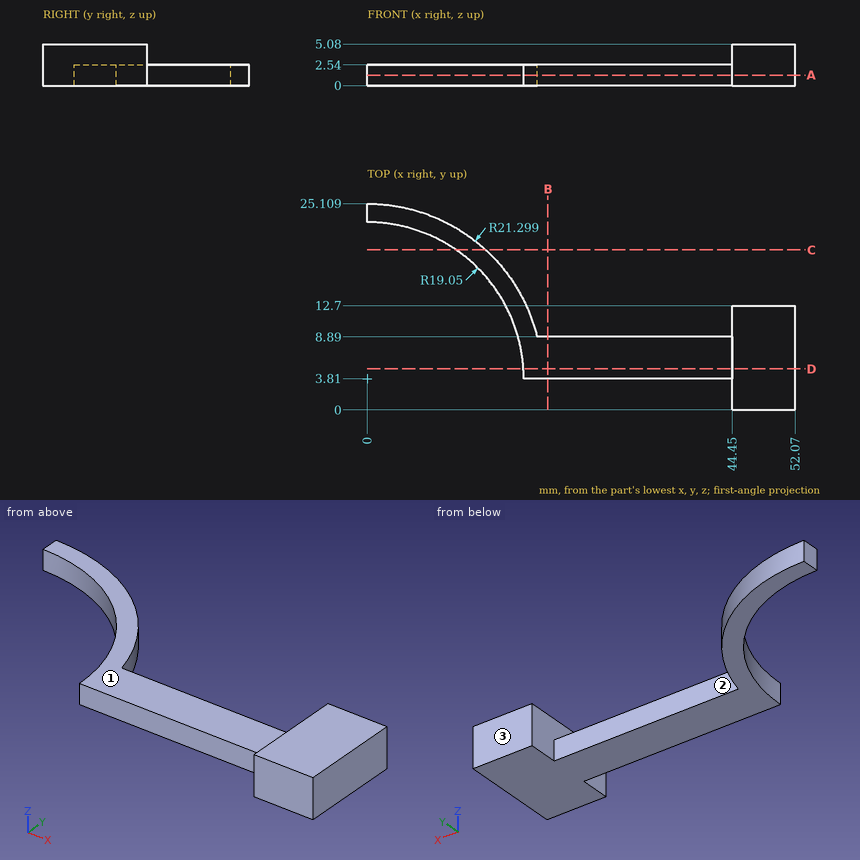
The figure shows three views and two pictorial views of one solid part (mm, origin at its lowest corner). Answer the questions. A direction names the side the tool comes from. Coordinates: 2 decimals unless noted, no trailing zeros. Loops run counter-clockwise (first coordinate to the right, second up) from the corner with the lowest first, then second, coordinate; pieces in that order, holes last. Notation, with made-up numbers: M 71.5,35 L 85.5,35 A31 ccw 85.5,59 Z; hole C 66,-32 d8. An arc over 180 degrees is marked long. Use CSV: the item, a comma, the result in double quotes. Start each with the question number.
(1) Given pin 1 Ø1.3 at (x, z) = (38, 2) entering from -Y; pin 2 Ø1 at (y, z) = (14, 2.5) entering from -X; pin 3 Ø3 at (y, z) = (21, 2) entering from +X (1 decimal), each flat-ended and moving along its own axis, determine where each tip first touches the part or whether it passes through.
(2) Find section C-C, the plane y = 19.5. Give the vertices of the cut face in (x, z).
(3) For the marked faces 1, 2 and 3, determine the directions among +Z, -Z, +X, -X, +Y, -Y from which every point of the face is accessible in a straight line to the end or side of a thin tool.
(4) Consider line 1 (Y direction, x = 35, z = 0.35); line 2 (X direction, y = 11.75, z = 4.1); line 3 (Z direction, x = 31.5, y = 8.5). Determine where each line is inside the solid, lowest interval first.
(5) Find section B-B, the plane x = 22. Give the vertices of the cut face in (y, z).
(6) Find section A-A, the plane z = 1.3. Give the vertices of the cut face in (x, y), then the cut area to 3 significant figures.
(7) Find section D-D, the plane y = 5. Give the vertices of the cut face in (x, z).
Recorded:
1,pin 1,"stops at y = 3.81"
1,pin 2,"stops at x = 15.77"
1,pin 3,"stops at x = 14.4"
2,outline,"M 10.8,0 L 14.4,0 L 14.4,2.54 L 10.8,2.54 Z"
3,face 1,"+Z, -X, +Y, -Y"
3,face 2,"+Z, -Z, +Y"
3,face 3,"+Z, -Z, +X, +Y"
4,line 1,"y = 3.81 to 8.89"
4,line 2,"x = 44.45 to 52.07"
4,line 3,"z = 0 to 2.54"
5,outline,"M 3.81,0 L 8.89,0 L 8.89,2.54 L 3.81,2.54 Z"
6,outline,"M 0,22.86 A19.05 cw 19.05,3.81 L 44.45,3.81 L 44.45,0 L 52.07,0 L 52.07,12.7 L 44.45,12.7 L 44.45,8.89 L 20.68,8.89 A21.3 ccw 0,25.11 Z"
6,area,"287 mm^2"
7,outline,"M 19.01,0 L 52.07,0 L 52.07,5.08 L 44.45,5.08 L 44.45,2.54 L 19.01,2.54 Z"
